Verification items for this drawing (mm, ordinates from the low corner). Round coordinates to 2 decimals unless told otherwise and drop trailing zeros. Write each loop counter-clockwise with the first axis right and the second up, starting at its lowest first coordinate (ties: lowest second). Pieces come first, ordered by that corner, then holes. Notation, with made-up numbers: (76, 13) -> (95, 13) arc R18 ccw to (95, 26) -> close; hole circle Ø9 at (-0.5, -17). An arc over 180 degrees is marked (long way). One line per question, with ' | ' between items.
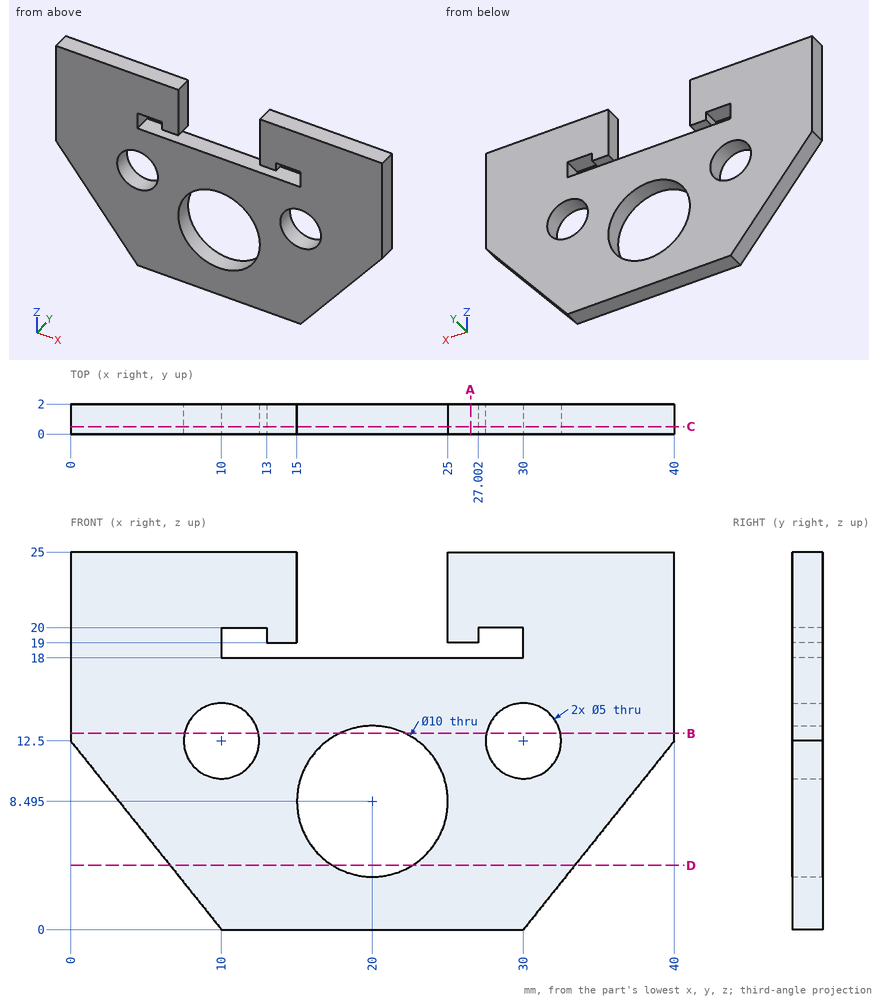
(1) Sectioned sample at C-C on y = 0.5. Record the cut outline in (x, z) (1 decimal), then the cut area to 3 significant figures.
Resolved:
outline: (0, 12.5) -> (10, 0) -> (30, 0) -> (40, 12.5) -> (40, 25) -> (25, 25) -> (25, 19) -> (27, 19) -> (27, 20) -> (30, 20) -> (30, 18) -> (10, 18) -> (10, 20) -> (13, 20) -> (13, 19) -> (15, 19) -> (15, 25) -> (0, 25) -> close; hole circle Ø5 at (10, 12.5); hole circle Ø10 at (20, 8.5); hole circle Ø5 at (30, 12.5) | area: 671 mm2
(2) Go/stop test with a flat-tipped pin: pin 1 (0.6 mm diameter, centred on x = 29, y = 1, fed in from -Z). Record where the tip stops, or that it passes through.
Resolved:
pin 1: stops at z = 0
(3) Material ranges on line 1 (X direction, y = 0.85, z = 14); line 2 (Z direction, x = 11, y = 0.5); line 3 (X direction, y = 0.75, z = 11.5) (1 decimal), recorded low to high.
Resolved:
line 1: x = 0 to 8, 12 to 28, 32 to 40 | line 2: z = 0 to 10.21, 14.79 to 18, 20 to 25 | line 3: x = 0.8 to 7.7, 12.3 to 16, 24 to 27.7, 32.3 to 39.2
(4) Sectioned sample at B-B on z = 13. Record the cut outline in (x, y).
Resolved:
outline: (0, 0) -> (7.55, 0) -> (7.55, 2) -> (0, 2) -> close; (12.45, 0) -> (17.83, 0) -> (17.83, 2) -> (12.45, 2) -> close; (22.17, 0) -> (27.55, 0) -> (27.55, 2) -> (22.17, 2) -> close; (32.45, 0) -> (40, 0) -> (40, 2) -> (32.45, 2) -> close
(5) Sectioned sample at A-A on x = 26.5. Record the cut outline in (y, z).
Resolved:
outline: (0, 0) -> (2, 0) -> (2, 18) -> (0, 18) -> close; (0, 19) -> (2, 19) -> (2, 25) -> (0, 25) -> close
(6) Sectioned sample at D-D on z = 4.25. Record the cut outline in (x, y).
Resolved:
outline: (6.6, 0) -> (17.36, 0) -> (17.36, 2) -> (6.6, 2) -> close; (22.64, 0) -> (33.4, 0) -> (33.4, 2) -> (22.64, 2) -> close
